from build123d import *

# Parameters (mm, degrees)
ESQUISSE1_W        = 60
ESQUISSE1_H        = 35
ESQUISSE1_R        = 6
ESQUISSE1_R_2      = 4
BOSS_EXTRU_1_DEPTH = 25
CONG_1_R           = 10


with BuildPart() as part:
    # Esquisse1 → Boss.-Extru.1 (new body)
    with BuildSketch(Plane.XY):
        with Locations((30, 17.5)):
            Rectangle(ESQUISSE1_W, ESQUISSE1_H)
        with Locations((30, 17.5)):
            Circle(ESQUISSE1_R, mode=Mode.SUBTRACT)
        with Locations((47.275578018, 27.57742051)):
            Circle(ESQUISSE1_R_2, mode=Mode.SUBTRACT)
        with Locations(Location((12.724421982, 7.42257949, 0), (0, 0, 180))):
            Circle(ESQUISSE1_R_2, mode=Mode.SUBTRACT)
    extrude(amount=BOSS_EXTRU_1_DEPTH)

    # Congé1
    cong_1_edges = [part.edges().sort_by_distance(p)[0] for p in [
        (0, 35, 12.5),
        (60, 35, 12.5),
        (60, 0, 12.5),
        (0, 0, 12.5),
    ]]
    fillet(cong_1_edges, radius=CONG_1_R)


solid = part.part
Design review of the part built by this model. Coordinates are the model's own, in mm. Give positions to 0.01 mm unless a question says otherwise; leave off trailing zeros. Write each loop counter-clockwise with the first axis right and the second up, starting at its lowest first coordinate (ties: lowest second). Pieces come first, ordered by that corner, then holes. Notation, with made-up numbers: M 46.5,34.5 L 67.5,34.5 A26 cw 67.5,56.5 Z; hole C 41.25,75.5 d5. An arc over 180 degrees is marked long. Answer as a JSON object with one key per item and string values. Group by question number.
1) We need section A-A (x = 30). Give the boundary of the cut face in (y, z), and give its area (3 significant figures).
2) We need section D-D (y = 2). Give the boundary of the cut face in (x, z), and give its area (3 significant figures).
3) Mouldability with a two-part tool opening along Y and no side actions: class faces 1 (the face through (44.101, 25.143, 12.325)), 2 (the face through (30, 35, 12)), 3 (the face through (0, 17, 12)) as released by +Y, released by -Y, zero draft, split by the parting line, or undercut.
4) We need section C-C (z = 13). Give the boundary of the cut face in (x, y).
5) For line 1 along X through (y, z) = (28.5, 15.5); line 2 along Y through (x, z) = (49, 23.5); line 3 along Y through (x, z) = (16, 11.5), list the stretches that pass through material, from the lowest coordinate up.
6) Clearance check with flat-ended pins moving along their axes: pin 1 Ø6.5 at (x, y) = (47.28, 27.58) entering from -Z; pin 2 Ø1 at (y, z) = (30, 21.5) entering from -X. State where each tip first meets the part, or that it passes through.
7) We need section B-B (y = 8.5). Give the boundary of the cut face in (x, z), and give its area (3 significant figures).
Answer key:
{
 "1": {"outline": "M 0,0 L 11.5,0 L 11.5,25 L 0,25 Z; M 23.5,0 L 35,0 L 35,25 L 23.5,25 Z", "area": "575 mm²"},
 "2": {"outline": "M 4,0 L 56,0 L 56,25 L 4,25 Z", "area": "1,300 mm²"},
 "3": {"face 1": "undercut", "face 2": "released by +Y", "face 3": "zero draft"},
 "4": {"outline": "M 0,10 A10 ccw 10,0 L 50,0 A10 ccw 60,10 L 60,25 A10 ccw 50,35 L 10,35 A10 ccw 0,25 Z; hole C 12.72,7.42 d8; hole C 30,17.5 d12; hole C 47.28,27.58 d8"},
 "5": {"line 1": "x = 0.63 to 43.38, 51.17 to 59.37", "line 2": "y = 0 to 23.97, 31.19 to 35", "line 3": "y = 0 to 5.13, 9.72 to 35"},
 "6": {"pin 1": "passes through", "pin 2": "stops at x = 1.07"},
 "7": {"outline": "M 0.11,0 L 8.87,0 L 8.87,25 L 0.11,25 Z; M 16.58,0 L 59.89,0 L 59.89,25 L 16.58,25 Z", "area": "1,300 mm²"}
}
